```python
from build123d import *

# Parameters (mm, degrees)
SKETCH_1_W      = 20
SKETCH_1_H      = 180
SKETCH_1_R      = 5
EXTRUDE_1_DEPTH = 15
FILLET_1_R      = 10


with BuildPart() as part:
    # 草图1 → 凸台-拉伸1 (new body)
    with BuildSketch(Plane.XY):
        Rectangle(SKETCH_1_W, SKETCH_1_H)
        with Locations((0, -80)):
            Circle(SKETCH_1_R, mode=Mode.SUBTRACT)
        with Locations(Location((0, 80, 0), (0, 0, 180))):
            Circle(SKETCH_1_R, mode=Mode.SUBTRACT)
        Circle(SKETCH_1_R, mode=Mode.SUBTRACT)
        with Locations((0, -40)):
            Circle(SKETCH_1_R, mode=Mode.SUBTRACT)
        with Locations((0, 40)):
            Circle(SKETCH_1_R, mode=Mode.SUBTRACT)
    extrude(amount=EXTRUDE_1_DEPTH)

    # 圆角1
    fillet_1_edges = [part.edges().sort_by_distance(p)[0] for p in [
        (-10, -90, 7.5),
        (10, -90, 7.5),
        (10, 90, 7.5),
        (-10, 90, 7.5),
    ]]
    fillet(fillet_1_edges, radius=FILLET_1_R - 0.0001)  # a hair under: the kernel refuses the full size


solid = part.part
```
CAD build for the part. Positions are in the model's coordinates, mm. Give positions to 0.01 mm unless a question says otherwise; leave off trailing zeros. Write each loop counter-clockwise with the first axis right and the second up, starting at its lowest first coordinate (ties: lowest second). Pieces come first, ordered by that corner, then holes. Notation, with made-up numbers: M 7.25,7 L 28.25,7 A30 cw 28.25,44 Z; hole C 66.5,-33 d11. An arc over 180 degrees is marked long. Return JSON: item names as keys, results as strings. Group by question number.
(1) Flat gauge pins, fed straight in: pin 1 Ø11.5 at (x, y) = (0, 0) entering from +Z; pin 2 Ø1 at (x, z) = (1, 2.5) entering from +Y. Where does each tip first touch, or does it go through?
(2) Band-saw the part on A-A (z = 12.25). State how many separate pieces and enclosed holes the cut face has, and give its area (3 significant figures).
(3) Band-saw the part on C-C (x = -7.5). Give the cut face in (y, z).
(4) Mould opens along Y. For faces 1 (the face through (-7.15, 86.99, 7.6)), 2 (the face through (3, -36, 7)), 3 (the face through (7, 1, 15)), 4 (the face through (6.99, -87.15, 7.6)) say: pulls with the +Y half, pulls with the -Y half, needs draft (parallel to the pull), parting line crosses it, or undercut.
(5) Band-saw the part on B-B (y = -40). Give the cut face in (x, z).
(6) Drill centre lines: L1, parallel to Y at x = 0, z = 10.25; L2, parallel to Y at x = 1.5, z = 3.25; L3, parallel to X at y = 80, z = 7.75. Where is each one in solid material? Low to high. Write a range as [from, to].
Entries:
{
 "1": {"pin 1": "stops at z = 15", "pin 2": "stops at y = 89.99"},
 "2": {"separate pieces": "1", "enclosed holes": "5", "area": "3,120 mm^2"},
 "3": {"outline": "M -86.61,0 L 86.61,0 L 86.61,15 L -86.61,15 Z"},
 "4": {"face 1": "pulls with the +Y half", "face 2": "undercut", "face 3": "needs draft", "face 4": "pulls with the -Y half"},
 "5": {"outline": "M -10,0 L -5,0 L -5,15 L -10,15 Z; M 5,0 L 10,0 L 10,15 L 5,15 Z"},
 "6": {"L1": "y = [-90, -85], [-75, -45], [-35, -5], [5, 35], [45, 75], [85, 90]", "L2": "y = [-89.89, -84.77], [-75.23, -44.77], [-35.23, -4.77], [4.77, 35.23], [44.77, 75.23], [84.77, 89.89]", "L3": "x = [-10, -5], [5, 10]"}
}
